```python
from build123d import *

# Parameters (mm, degrees)
EXTRUDE_1_DEPTH = 300


with BuildPart() as part:
    # уголок-20х20 → Бобышка-Вытянуть1 (new body)
    with BuildSketch(Plane(origin=(0, 0, 0), x_dir=(1, 0, 0), z_dir=(0, 1, 0))):
        with BuildLine():
            Line((-10.917874396, 0.2), (-10.917874396, 19.8))
            ThreePointArc((-10.917874396, 19.8), (-10.859295752, 19.941421356), (-10.717874396, 20))
            Line((-10.717874396, 20), (-9.917874396, 20))
            ThreePointArc((-9.917874396, 20), (-9.77645304, 19.941421356), (-9.717874396, 19.8))
            Line((-9.717874396, 19.8), (-9.717874396, 1.4))
            ThreePointArc((-9.717874396, 1.4), (-9.659295752, 1.258578644), (-9.517874396, 1.2))
            Line((-9.517874396, 1.2), (8.882125604, 1.2))
            ThreePointArc((8.882125604, 1.2), (9.02354696, 1.141421356), (9.082125604, 1))
            Line((9.082125604, 1), (9.082125604, 0.2))
            ThreePointArc((9.082125604, 0.2), (9.02354696, 0.058578644), (8.882125604, 0))
            Line((8.882125604, 0), (-10.717874396, 0))
            ThreePointArc((-10.717874396, 0), (-10.859295752, 0.058578644), (-10.917874396, 0.2))
        make_face()
    extrude(amount=EXTRUDE_1_DEPTH)


solid = part.part
```
Check sheet for the modelled part. Datum: model origin and axes. Units: mm. A direction names the side the tool comes from. Give positions to 0.01 mm unless a question says otherwise; leave off trailing zeros. Loops run counter-clockwise (first coordinate to the right, second up) from the corner with the lowest first, then second, coordinate; pieces in that order, holes last. Notation, with made-up numbers: M 61,-23.5 L 79,-23.5 A29 cw 79,9.5 Z; hole C 50.25,75.25 d5. An arc over 180 degrees is marked long. Answer in a Markdown table with one row per item.
1) Tool access check on faces 1 (the face through (-1, 148, 0)), 2 (the face through (0, 148, -1.2)). Record the directions out of +Z, -Z, +X, -X, +Y, -Y that give a thin tool (end or side, any length) a straight path to the whole face; none if there is none.
Solutions:
| item | result |
|---|---|
| face 1 | +Z, +X, -X, +Y, -Y |
| face 2 | -Z, +X, +Y, -Y |
2) Cross-section at C-C (x = -1.25). Enter the section's corners in (y, z).
Solutions:
| item | result |
|---|---|
| outline | M 0,-1.2 L 300,-1.2 L 300,0 L 0,0 Z |
3) Depth check by flat-ended pin: pin 1 (3 mm diameter, centred on x = 6, y = 191, fed in from -Z); pin 2 (9 mm diameter, centred on y = 152.5, z = -7, fed in from +X). Enter the tip coordinate at first touch or a pass-through.
Solutions:
| item | result |
|---|---|
| pin 1 | stops at z = -1.2 |
| pin 2 | stops at x = -9.72 |
4) Thickness scan on line 1 (Z direction, x = 3, y = 16); line 2 (X direction, y = 168, z = -4.5). Record the ranges inside material, lowest first.
Solutions:
| item | result |
|---|---|
| line 1 | z = -1.2 to 0 |
| line 2 | x = -10.92 to -9.72 |
5) Cross-section at B-B (z = -15.75). Enter the section's corners in (x, y), plus the area to 3 significant figures.
Solutions:
| item | result |
|---|---|
| outline | M -10.92,0 L -9.72,0 L -9.72,300 L -10.92,300 Z |
| area | 360 mm^2 |
6) Cross-section at A-A (y = 145.5). Enter the section's corners in (x, z), plus the area to 3 significant figures.
Solutions:
| item | result |
|---|---|
| outline | M -10.92,-19.8 A0.2 ccw -10.72,-20 L -9.92,-20 A0.2 ccw -9.72,-19.8 L -9.72,-1.4 A0.2 cw -9.52,-1.2 L 8.88,-1.2 A0.2 ccw 9.08,-1 L 9.08,-0.2 A0.2 ccw 8.88,0 L -10.72,0 A0.2 ccw -10.92,-0.2 Z |
| area | 46.5 mm^2 |
